Read the model definition and answer for the solid it produces. Units are mm, in the model's axes. Face numbers are marked on the shaded views. A direction names the side the tool comes from. Round coordinates to 2 decimals unless told otherwise and drop trailing zeros. Order: outer loops, then holes, each group sorted by start corner. A loop starts at its lowest first (then second) coordinate and runs counter-clockwise, first axis right, second up.
from build123d import *

# Parameters (mm, degrees)
PAD003_DEPTH    = 34
FILLET001_R     = 5
FILLET002_R     = 10
FILLET003_R     = 5
SKETCH013_R     = 2
POCKET005_DEPTH = 5


with BuildPart() as part:
    # Sketch009 (on XY_Plane001 of Origin002) → Pad003 (new body)
    with BuildSketch(Plane.XY.offset(1)):
        Polygon((0, 20), (0, -20), (-80, -70), (-95, -70), (-95, -65), (-80, -65), (-5, -18.125), (-5, 18.125), (-80, 65), (-95, 65), (-95, 70), (-80, 70), align=None)
    extrude(amount=PAD003_DEPTH)

    # Fillet001
    fillet001_edges = [part.edges().sort_by_distance(p)[0] for p in [
        (-95, -67.5, 35),
        (-95, 67.5, 35),
    ]]
    fillet(fillet001_edges, radius=FILLET001_R)

    # Fillet002
    fillet002_edges = [part.edges().sort_by_distance(p)[0] for p in [
        (-80, -70, 18),
        (0, -20, 18),
        (0, 20, 18),
        (-80, 70, 18),
    ]]
    fillet(fillet002_edges, radius=FILLET002_R)

    # Fillet003
    fillet003_edges = [part.edges().sort_by_distance(p)[0] for p in [
        (-80, -65, 18),
        (-5, -18.125, 18),
        (-80, 65, 18),
        (-5, 18.125, 18),
    ]]
    fillet(fillet003_edges, radius=FILLET003_R)

    # Sketch013 (on Face10 of Fillet003) → Pocket005 (cut)
    with BuildSketch(Plane(origin=(8.9887640449, 14.3820224719, 0), x_dir=(-0.847998304, 0.52999894, 0), z_dir=(0.52999894, 0.847998304, 0))):
        with Locations((60, 5)):
            Circle(SKETCH013_R)
    extrude(amount=-POCKET005_DEPTH, mode=Mode.SUBTRACT)


solid = part.part
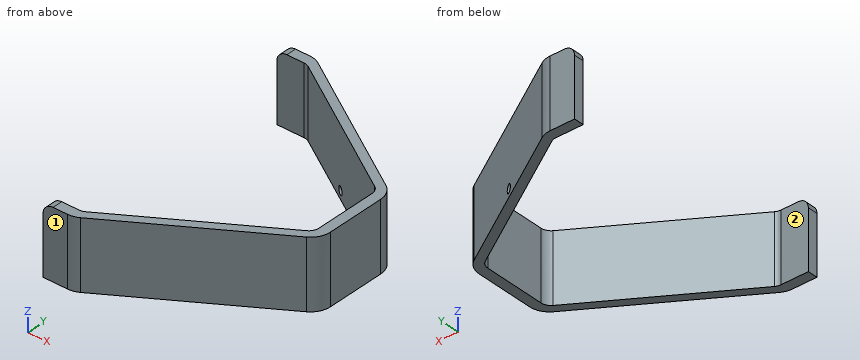
Q1. A cutting plane is placed at C-C, the plane y = 53.5. Give the vertices of the cut face in (x, z), plus the area to 3 significant figures.
Outcome:
outline: (-61.6, 1) - (-53.6, 1) - (-53.6, 35) - (-61.6, 35) - close
area: 272 mm2
Q2. A cutting plane is placed at B-B, the plane z = 22. Give the vertices of the cut face in (x, y).
Outcome:
outline: (-95, -70) - (-82.87, -70) arc R10 ccw to (-77.57, -68.48) - (-4.7, -22.94) arc R10 ccw to (0, -14.46) - (0, 14.46) arc R10 ccw to (-4.7, 22.94) - (-77.57, 68.48) arc R10 ccw to (-82.87, 70) - (-95, 70) - (-95, 65) - (-81.43, 65) arc R5 cw to (-78.78, 64.24) - (-7.35, 19.59) arc R5 cw to (-5, 15.35) - (-5, -15.35) arc R5 cw to (-7.35, -19.59) - (-78.78, -64.24) arc R5 cw to (-81.43, -65) - (-95, -65) - close
Q3. A cutting plane is placed at D-D, the plane z = 32. Give the vertices of the cut face in (x, y).
Outcome:
outline: (-94.58, -70) - (-82.87, -70) arc R10 ccw to (-77.57, -68.48) - (-4.7, -22.94) arc R10 ccw to (0, -14.46) - (0, 14.46) arc R10 ccw to (-4.7, 22.94) - (-77.57, 68.48) arc R10 ccw to (-82.87, 70) - (-94.58, 70) - (-94.58, 65) - (-81.43, 65) arc R5 cw to (-78.78, 64.24) - (-7.35, 19.59) arc R5 cw to (-5, 15.35) - (-5, -15.35) arc R5 cw to (-7.35, -19.59) - (-78.78, -64.24) arc R5 cw to (-81.43, -65) - (-94.58, -65) - close
Q4. Straight lines are drawn through the part: probe 1 along X at (y, z) = (7.5, 7); probe 2 along Y at (x, z) = (-33.5, 21); probe 3 along Y at (x, z) = (-69, 3) (3 decimals). For each, find the intervals that lie inside material, in ascending order.
Outcome:
probe 1: x = -5 to 0
probe 2: y = -40.94 to -35.94, 35.94 to 40.94
probe 3: y = -63.125 to -58.125, 58.125 to 63.125
Q5. A cutting plane is placed at A-A, the plane x = -11. Give the vertices of the cut face in (y, z) (3 decimals).
Outcome:
outline: (-26.875, 1) - (-21.875, 1) - (-21.875, 35) - (-26.875, 35) - close; (21.875, 1) - (26.875, 1) - (26.875, 35) - (21.875, 35) - close
Q6. For the marked faces 1 and 2, determine the directions among +Z, -Z, +X, -X, +Y, -Y from which every point of the face is accessible in a straight line to the end or side of a thin tool.
Outcome:
face 1: +Z, -Z, +X, -X, -Y
face 2: +Z, -Z, -X
Q7. Flat-ended cylindrical pins translate along their axes: pin 1 (2 mm diameter, centred on y = 12, z = 8.5, fed in from -X); pin 2 (2 mm diameter, centred on y = -23.5, z = 5, fed in from +X); pin 3 (3 mm diameter, centred on y = 18, z = 15, fed in from -X). Find the tip coordinate at first contact, or state that the pin passes through.
Outcome:
pin 1: stops at x = -5
pin 2: stops at x = -4.06
pin 3: stops at x = -7.21
